Part model, mm, in its own coordinate system. A direction names the side the tool comes from. Round coordinates to 2 decimals unless told otherwise and drop trailing zeros. Loops run counter-clockwise (first coordinate to the right, second up) from the corner with the lowest first, then second, coordinate; pieces in that order, holes last. Notation, with made-up numbers: M 59,50 L 114,50 A21 cw 114,87 Z; hole C 2.5,-22 d11. An arc over 180 degrees is marked long. Put each result on its own line as item: value. Start each with the question number.
1) Slice it at D-D on x = 19.5. Give the cut face in (y, z), then the cut area to 3 significant figures.
2) Which spindle directions (+Z, -Z, +X, -X, +Y, -Y) get a long thin tool onto all of the face, cutting with end or side? Do faces 1 (the flat face through (9, 9, 3)), 2 (the flat face through (10, 2, 6)), 3 (the flat face through (11, 12, 6)), 4 (the flat face through (10, 7, 0)), 5 (the flat face through (20, 2, 3)). Say none if no direction does.
3) Probe line 1 along Y through (x, z) = (9.3, 5.2); line 2 along Y through (x, z) = (9.5, 0.5); line 3 along X through (y, z) = (4.75, 0.75). List the from-to ranges inside material, lowest first.
4) Pull direction Y, two halves, no side cores. Call faces 6 (the cylindrical face through (7.776, 10.368, 4.521)), 7 (the flat face through (-1, 11, 3)), 8 (the cylindrical face through (12.066, 11.871, 1.479)), 9 (the flat face through (-2.7, 8, 3)): +Y half, -Y half, draft (parallel to the pull), parting line (faces both ways), or undercut.
5) Slice it at B-B on z = 0.75. Give the cut face in (x, y).
6) Slice it at C-C on y = 10. Give the cut face in (x, z), then the cut area to 3 significant figures.
7) Slice it at A-A on x = 9.3. Give the cut face in (y, z), then the cut area to 3 significant figures.
8) Drop flat-ended pins along their axis: pin 1 Ø1 at (x, y) = (9, 15.5) entering from +Z; pin 2 Ø2 at (x, y) = (9.3, 11) entering from +Z; pin 3 Ø3 at (y, z) = (9.5, 4.5) entering from +X; pin 4 Ø7 at (x, y) = (14.5, 13.5) entering from -Z. Give the stop position or say it passes through.
```python
from build123d import *

# Parameters (mm, degrees)
SKETCH1_R           = 2.9
BOSS_EXTRUDE1_DEPTH = 6
BOSS_EXTRUDE2_DEPTH = 26.3
BOSS_EXTRUDE3_DEPTH = 6
SKETCH5_R           = 2.9
SKETCH5_R_2         = 1.65
BOSS_EXTRUDE4_DEPTH = 3


with BuildPart() as part:
    # Sketch1 → Boss-Extrude1 (new body)
    with BuildSketch(Plane.XY):
        with BuildLine():
            Line((0, 0), (20, 0))
            Line((20, 0), (20, 4))
            Line((20, 4), (23.6, 4))
            Line((23.6, 4), (23.6, 11))
            Line((23.6, 11), (17.3, 11))
            ThreePointArc((17.3, 11), (9.3, 19), (1.3, 11))
            Line((1.3, 11), (-2.7, 11))
            Line((-2.7, 11), (-2.7, 4))
            Line((-2.7, 4), (0, 4))
            Line((0, 4), (0, 0))
        make_face()
        with Locations((9.3, 11)):
            Circle(SKETCH1_R, mode=Mode.SUBTRACT)
    extrude(amount=BOSS_EXTRUDE1_DEPTH)

    # Sketch2 → Boss-Extrude2 (add)
    with BuildSketch(Plane.ZY.offset(2.7)):
        with BuildLine():
            Line((6, 4), (6, 5))
            ThreePointArc((6, 5), (6.292893219, 4.292893219), (7, 4))
            Line((7, 4), (6, 4))
        make_face()
        with BuildLine():
            Line((0, 4), (-1, 4))
            ThreePointArc((-1, 4), (-0.292893219, 4.292893219), (0, 5))
            Line((0, 5), (0, 4))
        make_face()
    extrude(amount=-BOSS_EXTRUDE2_DEPTH)

    # Sketch4 → Boss-Extrude3 (add)
    with BuildSketch(Plane.XY.offset(6)):
        with BuildLine():
            Line((23.1, 4), (23.1, 5))
            ThreePointArc((23.1, 5), (23.392893219, 4.292893219), (24.1, 4))
            Line((24.1, 4), (23.1, 4))
        make_face()
        with BuildLine():
            Line((-1.5, 4), (-2.5, 4))
            ThreePointArc((-2.5, 4), (-1.792893219, 4.292893219), (-1.5, 5))
            Line((-1.5, 5), (-1.5, 4))
        make_face()
    extrude(amount=-BOSS_EXTRUDE3_DEPTH)

    # Sketch5 → Boss-Extrude4 (add)
    with BuildSketch(Plane(origin=(0, 0, 6), x_dir=(-1, 0, 0), z_dir=(0, 0, -1))):
        with Locations((-9.3, 11)):
            Circle(SKETCH5_R)
        with Locations((-9.3, 11)):
            Circle(SKETCH5_R_2, mode=Mode.SUBTRACT)
    extrude(amount=BOSS_EXTRUDE4_DEPTH)


solid = part.part
```
Recorded:
1. outline: M 0,0 L 4,0 L 4,-1 A1 cw 5,0 L 11,0 L 11,6 L 5,6 A1 cw 4,7 L 4,6 L 0,6 Z
1. area: 66.4 mm2
2. face 1: -Z
2. face 2: +Z, +X, -X, -Y
2. face 3: +Z, +X, -X, +Y
2. face 4: -Z, +X, -X, +Y
2. face 5: +Z, -Z, +X, -Y
3. line 1: y = 0 to 9.35, 12.65 to 19
3. line 2: y = 0 to 8.11, 13.89 to 19
3. line 3: x = -2.7 to 23.6
4. face 6: undercut
4. face 7: +Y half
4. face 8: undercut
4. face 9: draft
5. outline: M -2.7,4 L 0,4 L 0,0 L 20,0 L 20,4 L 24.1,4 A1 cw 23.6,4.13 L 23.6,11 L 17.3,11 A8 ccw 1.3,11 L -2.7,11 Z; hole C 9.3,11 d5.8
6. outline: M -2.7,0 L 6.58,0 L 6.58,3 L 7.99,3 L 7.99,6 L -2.7,6 Z; M 10.61,3 L 12.02,3 L 12.02,0 L 23.6,0 L 23.6,6 L 10.61,6 Z
6. area: 134 mm2
7. outline: M 0,0 L 4,0 L 4,-1 A1 cw 5,0 L 8.1,0 L 8.1,3 L 9.35,3 L 9.35,6 L 5,6 A1 cw 4,7 L 4,6 L 0,6 Z; M 12.65,3 L 13.9,3 L 13.9,0 L 19,0 L 19,6 L 12.65,6 Z
7. area: 87.1 mm2
8. pin 1: stops at z = 6
8. pin 2: passes through
8. pin 3: stops at x = 23.6
8. pin 4: stops at z = 0
